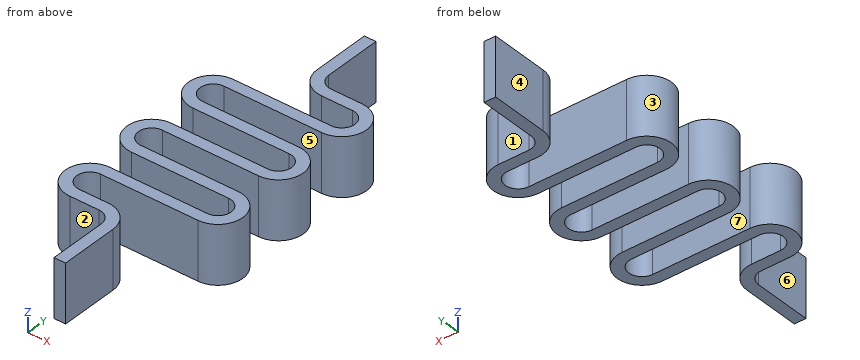
```python
from build123d import *

# Parameters (mm, degrees)
PAD_DEPTH = 10


with BuildPart() as part:
    # Sketch → Pad (new body)
    with BuildSketch(Plane.XY):
        with BuildLine():
            ThreePointArc((-8.268261, 24.087282), (-12.523239, 19.832304), (-8.268261, 15.577326))
            Line((8.472095, 15.577326), (-8.268261, 15.577326))
            ThreePointArc((8.472095, 11.06737), (10.727073, 13.322348), (8.472095, 15.577326))
            Line((-8.268261, 11.06737), (8.472095, 11.06737))
            ThreePointArc((-8.268261, 11.06737), (-12.523239, 6.812392), (-8.268261, 2.557415))
            Line((-3.254978, 2.557415), (-8.268261, 2.557415))
            ThreePointArc((-1, 0.302437), (-1.660468, 1.896947), (-3.254978, 2.557415))
            Line((-1, 0.302437), (-1, -9.697563))
            Line((1, -9.697563), (-1, -9.697563))
            Line((1, 0.302437), (1, -9.697563))
            ThreePointArc((1, 0.302437), (-0.246254, 3.31116), (-3.254978, 4.557415))
            Line((-8.268261, 4.557415), (-3.254978, 4.557415))
            ThreePointArc((-8.268261, 9.06737), (-10.523239, 6.812392), (-8.268261, 4.557415))
            Line((-8.268261, 9.06737), (8.472095, 9.06737))
            ThreePointArc((8.472095, 9.06737), (12.727073, 13.322348), (8.472095, 17.577326))
            Line((-8.268261, 17.577326), (8.472095, 17.577326))
            ThreePointArc((-8.268261, 22.087282), (-10.523239, 19.832304), (-8.268261, 17.577326))
            Line((-8.268261, 22.087282), (8.286925, 22.087282))
            ThreePointArc((8.286925, 22.087282), (12.541903, 26.34226), (8.286925, 30.597238))
            Line((-8.268261, 30.597238), (8.286925, 30.597238))
            ThreePointArc((-8.268261, 35.107193), (-10.523239, 32.852215), (-8.268261, 30.597238))
            Line((-8.268261, 35.107193), (8.568532, 35.107193))
            ThreePointArc((8.568532, 35.107193), (12.82351, 39.362171), (8.568532, 43.617149))
            Line((8.568532, 43.617149), (3.254978, 43.617149))
            ThreePointArc((1, 45.872127), (1.660468, 44.277617), (3.254978, 43.617149))
            Line((1, 55.872127), (1, 45.872127))
            Line((-1, 55.872127), (1, 55.872127))
            Line((-1, 45.872127), (-1, 55.872127))
            ThreePointArc((-1, 45.872127), (0.246254, 42.863403), (3.254978, 41.617149))
            Line((8.568532, 41.617149), (3.254978, 41.617149))
            ThreePointArc((8.568532, 37.107193), (10.82351, 39.362171), (8.568532, 41.617149))
            Line((-8.268261, 37.107193), (8.568532, 37.107193))
            ThreePointArc((-8.268261, 37.107193), (-12.523239, 32.852215), (-8.268261, 28.597238))
            Line((8.286925, 28.597238), (-8.268261, 28.597238))
            ThreePointArc((8.286925, 24.087282), (10.541903, 26.34226), (8.286925, 28.597238))
            Line((-8.268261, 24.087282), (8.286925, 24.087282))
        make_face()
    extrude(amount=PAD_DEPTH)


solid = part.part
```
The model under review builds one solid part; all positions refer to its coordinate system, in mm. Face numbers are marked on the shaded views. A direction names the side the tool comes from. Give positions to 0.01 mm unless a question says otherwise; leave off trailing zeros. Loops run counter-clockwise (first coordinate to the right, second up) from the corner with the lowest first, then second, coordinate; pieces in that order, holes last. Notation, with made-up numbers: (-29, -6.5) - (6, -6.5) arc R31 cw to (6, 22.5) - close; hole circle Ø1 at (-30.5, -11). An arc over 180 degrees is marked (long way). Answer as a JSON object with one key per item and string values.
Q1. Add section C-C on y = 40. State the section outline as (x, z) points.
Worked out:
{"outline": "(10.73, 0) - (12.78, 0) - (12.78, 10) - (10.73, 10) - close"}
Q2. Add section A-A on x = -7. State the section outline as (y, z) points, plus the area to 3 significant figures.
Worked out:
{"outline": "(2.56, 0) - (4.56, 0) - (4.56, 10) - (2.56, 10) - close; (9.07, 0) - (11.07, 0) - (11.07, 10) - (9.07, 10) - close; (15.58, 0) - (17.58, 0) - (17.58, 10) - (15.58, 10) - close; (22.09, 0) - (24.09, 0) - (24.09, 10) - (22.09, 10) - close; (28.6, 0) - (30.6, 0) - (30.6, 10) - (28.6, 10) - close; (35.11, 0) - (37.11, 0) - (37.11, 10) - (35.11, 10) - close", "area": "120 mm^2"}
Q3. For the marked faces 5, 6 and 7, list the 3-axis set-ups (+Z, -Z, +X, -X, +Y, -Y) from which the entire face can be reached by the end or side of a thin tool; tool diameter is ignored.
Worked out:
{"face 5": "+Z, -Z, +X", "face 6": "+Z, -Z, -X, -Y", "face 7": "+Z, -Z, -X"}
Q4. Add section B-B on y = 47. State the section outline as (x, z) points, plus the area to 3 significant figures.
Worked out:
{"outline": "(-1, 0) - (1, 0) - (1, 10) - (-1, 10) - close", "area": "20.0 mm^2"}
Q5. Insertion check: pin 1 (4 mm diameter, centred on x = 5.5, z = 7.5, fed in from +Y); pin 2 (5 mm diameter, centred on y = 49.5, z = 5, fed in from +X); pin 3 (5 mm diameter, centred on x = -1.5, z = 4.5, fed in from -Y); pin 4 (6 mm diameter, centred on x = 9, z = 5.5, fed in from -Y). Each pin has a flat end and moves straight along its axis. Give the tip position at first contact, or say it passes through.
Worked out:
{"pin 1": "stops at y = 43.62", "pin 2": "stops at x = 1", "pin 3": "stops at y = -9.7", "pin 4": "stops at y = 9.07"}
Q6. To check wall thickness, follow line 1 along Y through (x, z) = (4.75, 7.75); line 2 along Y through (x, z) = (-7.5, 5.5); line 3 along Y through (x, z) = (11.25, 9.25). State the ranges of each line that lie inside material, in increasing order.
Worked out:
{"line 1": "y = 9.07 to 11.07, 15.58 to 17.58, 22.09 to 24.09, 28.6 to 30.6, 35.11 to 37.11, 41.62 to 43.62", "line 2": "y = 2.56 to 4.56, 9.07 to 11.07, 15.58 to 17.58, 22.09 to 24.09, 28.6 to 30.6, 35.11 to 37.11", "line 3": "y = 10.1 to 16.55, 23.29 to 29.4, 36.06 to 42.67"}
Q7. Mouldability with a two-part tool opening along Y and no side actions: class the marked faces 1, 2, 3 and 4 as +Y half, -Y half, draft (parallel to the pull), parting line (faces both ways), or undercut.
Worked out:
{"face 1": "+Y half", "face 2": "-Y half", "face 3": "undercut", "face 4": "draft"}
